from build123d import *

# Parameters (mm, degrees)
SKETCH1_R                = 8.1
SKETCH1_R_2              = 7.1
BOSS_EXTRUDE1_DEPTH      = 1.3875
BOSS_EXTRUDE1_DEPTH_BACK = 14.4125
SKETCH3_R                = 1
CUT_EXTRUDE1_DEPTH       = 9.1
SKETCH4_R                = 0.5
CUT_EXTRUDE2_DEPTH       = 9.1000001


with BuildPart() as part:
    # Sketch1 → Boss-Extrude1 (new body, two sides)
    with BuildSketch(Plane.XY) as boss_extrude1_sk:
        Circle(SKETCH1_R)
        Circle(SKETCH1_R_2, mode=Mode.SUBTRACT)
    extrude(amount=BOSS_EXTRUDE1_DEPTH)
    extrude(boss_extrude1_sk.sketch, amount=-BOSS_EXTRUDE1_DEPTH_BACK)

    # Sketch3 → Cut-Extrude1 (cut, through all)
    with BuildSketch(Plane(origin=(0, 0, 0), x_dir=(0, 0, -1), z_dir=(1, 0, 0))):
        with Locations((1.440651468, 0)):
            Circle(SKETCH3_R)
    extrude(amount=-CUT_EXTRUDE1_DEPTH, mode=Mode.SUBTRACT)

    # Sketch4 → Cut-Extrude2 (cut, through all)
    with BuildSketch(Plane(origin=(0, 0, 0), x_dir=(1, 0, 0), z_dir=(0, 1, 0))):
        with Locations((0, 1.440651468)):
            Circle(SKETCH4_R)
    extrude(amount=CUT_EXTRUDE2_DEPTH, mode=Mode.SUBTRACT)


solid = part.part
Model file for the job. Use its own axes, mm. Round coordinates to 2 decimals unless told otherwise and drop trailing zeros. Order: outer loops, then holes, each group sorted by start corner. A loop starts at its lowest first (then second) coordinate and runs counter-clockwise, first axis right, second up.
(1) Band-saw the part on C-C (y = 6.5). List the corners of the cut face in (x, z), then the cut area to 3 significant figures.
(2) Drill centre lines: line 1 (X direction, y = 0, z = -4.75); line 2 (Y direction, x = 5, z = -3.5). Where is each one in solid material? Low to high.
(3) Band-saw the part on D-D (x = 3.5). List the corners of the cut face in (y, z).
(4) Band-saw the part on B-B (y = 0). List the corners of the cut face in (x, z).
(5) Band-saw the part on A-A (x = 0). List the corners of the cut face in (y, z), then the cut area to 3 significant figures.
(6) Pull direction X, two halves, no side cores. Call faces 1 (the face through (-0.065, 7.584, -1.936)), 2 (the face through (7.482, -3.102, -6.402)), 3 (the face through (-7.56, 0.04, -0.44)): released by +X, released by -X, zero draft, split by the parting line, or undercut.
(7) Pin check, flat tips, straight feed: pin 1 (6 mm diameter, centred on y = 6, z = -1, fed in from +X); pin 2 (1.5 mm diameter, centred on x = 4.5, y = -1.5, fed in from -Z); pin 3 (2 mm diameter, centred on y = -2, z = -11.5, fed in from -X); pin 4 (1.2 mm diameter, centred on y = 0, z = -1.44, fed in from -X). Stop position of each tip, or through.
Verdict:
1. outline: (-4.83, -14.41) - (-2.86, -14.41) - (-2.86, 1.39) - (-4.83, 1.39) - close; (2.86, -14.41) - (4.83, -14.41) - (4.83, 1.39) - (2.86, 1.39) - close
1. area: 62.5 mm2
2. line 1: x = -8.1 to -7.1, 7.1 to 8.1
2. line 2: y = -6.37 to -5.04, 5.04 to 6.37
3. outline: (-7.3, -14.41) - (-6.18, -14.41) - (-6.18, 1.39) - (-7.3, 1.39) - close; (6.18, -14.41) - (7.3, -14.41) - (7.3, 1.39) - (6.18, 1.39) - close
4. outline: (-8.1, -14.41) - (-7.1, -14.41) - (-7.1, -2.44) - (-8.1, -2.44) - close; (-8.1, -0.44) - (-7.1, -0.44) - (-7.1, 1.39) - (-8.1, 1.39) - close; (7.1, -14.41) - (8.1, -14.41) - (8.1, 1.39) - (7.1, 1.39) - close
5. outline: (-8.1, -14.41) - (-7.1, -14.41) - (-7.1, 1.39) - (-8.1, 1.39) - close; (7.1, -14.41) - (8.1, -14.41) - (8.1, -1.94) - (7.1, -1.94) - close; (7.1, -0.94) - (8.1, -0.94) - (8.1, 1.39) - (7.1, 1.39) - close
5. area: 30.6 mm2
6. face 1: undercut
6. face 2: split by the parting line
6. face 3: zero draft
7. pin 1: stops at x = 7.52
7. pin 2: passes through
7. pin 3: stops at x = -8.04
7. pin 4: stops at x = 7.07
